Source: three-view drawing plus pictorial views. Frame: mm from the lowest corner of the part. A direction names the side the tool comes from. Give positions to 0.01 mm unless a question says otherwise; leave off trailing zeros. Write each loop counter-clockwise with the first axis right and the second up, starting at its lowest first coordinate (ties: lowest second). Pieces come first, ordered by that corner, then holes. Notation, with made-up numbers: M 16.25,43 L 38.25,43 A26 ccw 38.25,59 Z; hole C 15.25,55.5 d5. An arc over 180 degrees is marked long. Return JSON: item names as keys, results as strings.
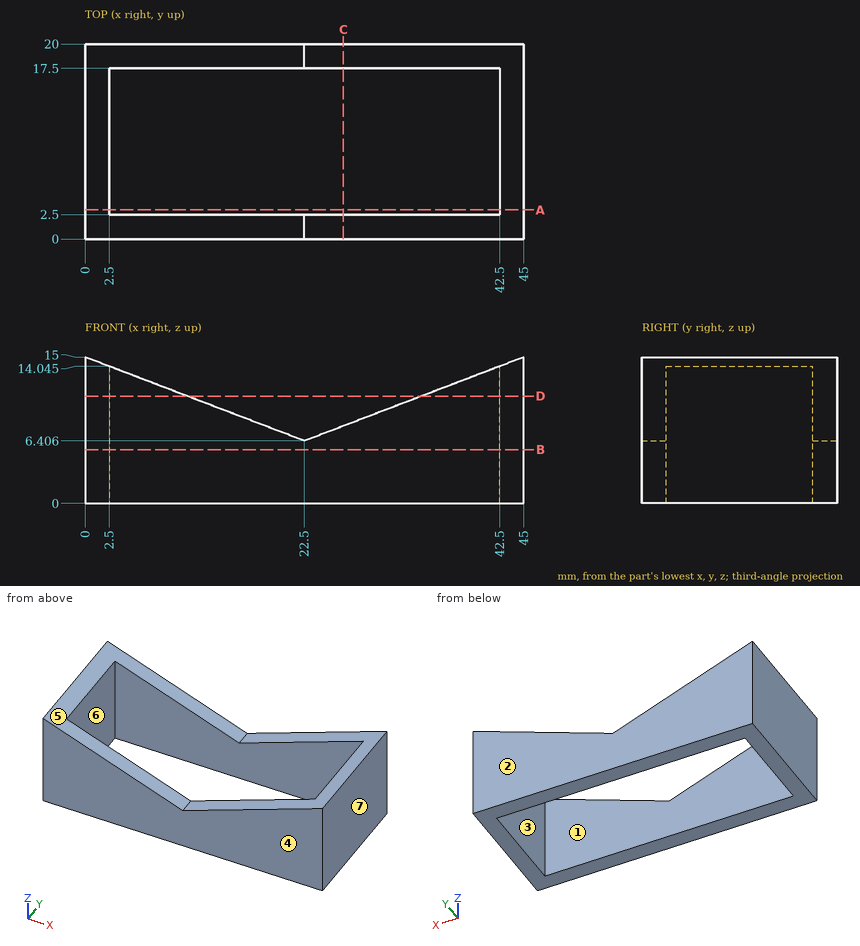
1) Draft query along Y for the marked faces 1, 2, 3 and 4. Return one class per face: released by +Y, released by -Y, zero draft, split by the parting line, or undercut.
Numbers:
{"face 1": "undercut", "face 2": "released by +Y", "face 3": "undercut", "face 4": "released by -Y"}
2) Line query: line 1 (Y direction, x = 7, z = 9.25); line 2 (X direction, y = 5.75, z = 0.5); line 3 (Z direction, x = 2, y = 1.5). Output: solid intervals per line, ascending. Write a range as [from, to].
Numbers:
{"line 1": "y = [0, 2.5], [17.5, 20]", "line 2": "x = [0, 2.5], [42.5, 45]", "line 3": "z = [0, 14.24]"}
3) Cut plane A-A, the plane y = 3. Return the cut outline in (x, z) (3 decimals), then the cut area to 3 significant figures.
Numbers:
{"outline": "M 0,0 L 2.5,0 L 2.5,14.045 L 0,15 Z; M 42.5,0 L 45,0 L 45,15 L 42.5,14.045 Z", "area": "72.6 mm²"}
4) Cut plane B-B, the plane z = 5.5. Return the cut outline in (x, y).
Numbers:
{"outline": "M 0,0 L 45,0 L 45,20 L 0,20 Z; hole M 2.5,2.5 L 42.5,2.5 L 42.5,17.5 L 2.5,17.5 Z"}
5) Contact query for flat-ended pins moving along their axis: pin 1 Ø5 at (x, y) = (33.5, 16.5) entering from +Z; pin 2 Ø1 at (x, y) = (33, 18) entering from +Z; pin 3 Ø1 at (x, y) = (23, 17.5) entering from +Z. Output: stop coordinate, or through.
Numbers:
{"pin 1": "stops at z = 11.48", "pin 2": "stops at z = 10.61", "pin 3": "stops at z = 6.79"}
6) Cut plane D-D, the plane z = 11. Return the cut outline in (x, y).
Numbers:
{"outline": "M 0,0 L 10.47,0 L 10.47,2.5 L 2.5,2.5 L 2.5,17.5 L 10.47,17.5 L 10.47,20 L 0,20 Z; M 34.53,0 L 45,0 L 45,20 L 34.53,20 L 34.53,17.5 L 42.5,17.5 L 42.5,2.5 L 34.53,2.5 Z"}
7) Set-up query: the marked faces 5, 6 and 7. Return all of +Z, -Z, +X, -X, +Y, -Y with unobstructed straight access to the full face (end or side cutting, diameter ignored); none if empty.
Numbers:
{"face 5": "+Z, +Y, -Y", "face 6": "+Z, -Z", "face 7": "+Z, -Z, +X, +Y, -Y"}
8) Cut plane C-C, the plane x = 26.5. Return the cut outline in (y, z).
Numbers:
{"outline": "M 0,0 L 2.5,0 L 2.5,7.93 L 0,7.93 Z; M 17.5,0 L 20,0 L 20,7.93 L 17.5,7.93 Z"}
